```python
from build123d import *

# Parameters (mm, degrees)
SKETCH1_R           = 2.5
BOSS_EXTRUDE1_DEPTH = 61.849
FILLET1_R           = 2
FILLET2_R           = 0.5


with BuildPart() as part:
    # Sketch1 → Boss-Extrude1 (new body, symmetric)
    with BuildSketch(Plane(origin=(0, 0, 0), x_dir=(0, 0, -1), z_dir=(1, 0, 0))):
        Polygon((-2.6, 10), (-2.6, 7.617766953), (-5.85, 7.617766953), (-1.832233047, 3.6), (1.832233047, 3.6), (5.85, 7.617766953), (2.6, 7.617766953), (2.6, 10), (10, 10), (10, 2.6), (7.617766953, 2.6), (7.617766953, 5.85), (3.6, 1.832233047), (3.6, -1.832233047), (7.617766953, -5.85), (7.617766953, -2.6), (10, -2.6), (10, -10), (2.6, -10), (2.6, -7.617766953), (5.85, -7.617766953), (1.832233047, -3.6), (-1.832233047, -3.6), (-5.85, -7.617766953), (-2.6, -7.617766953), (-2.6, -10), (-10, -10), (-10, -2.6), (-7.617766953, -2.6), (-7.617766953, -5.85), (-3.6, -1.832233047), (-3.6, 1.832233047), (-7.617766953, 5.85), (-7.617766953, 2.6), (-10, 2.6), (-10, 10), align=None)
        Circle(SKETCH1_R, mode=Mode.SUBTRACT)
    extrude(amount=BOSS_EXTRUDE1_DEPTH, both=True)

    # Fillet1
    fillet1_edges = [part.edges().sort_by_distance(p)[0] for p in [
        (0, 10, 10),
        (0, 10, -10),
        (0, -10, -10),
        (0, -10, 10),
    ]]
    fillet(fillet1_edges, radius=FILLET1_R)

    # Fillet2
    fillet2_edges = [part.edges().sort_by_distance(p)[0] for p in [
        (0, 10, 2.6),
        (0, 7.617766953, 5.85),
        (0, 3.6, 1.832233047),
        (0, 3.6, -1.832233047),
        (0, 7.617766953, -5.85),
        (0, 10, -2.6),
        (0, 2.6, -10),
        (0, 5.85, -7.617766953),
        (0, 1.832233047, -3.6),
        (0, -1.832233047, -3.6),
        (0, -5.85, -7.617766953),
        (0, -2.6, -10),
        (0, -10, -2.6),
        (0, -7.617766953, -5.85),
        (0, -3.6, -1.832233047),
        (0, -3.6, 1.832233047),
        (0, -7.617766953, 5.85),
        (0, -10, 2.6),
        (0, -2.6, 10),
        (0, -5.85, 7.617766953),
        (0, -1.832233047, 3.6),
        (0, 1.832233047, 3.6),
        (0, 5.85, 7.617766953),
        (0, 2.6, 10),
    ]]
    fillet(fillet2_edges, radius=FILLET2_R)


solid = part.part
```
Part model, mm, in its own coordinate system. A direction names the side the tool comes from. Round coordinates to 2 decimals unless told otherwise and drop trailing zeros. Loops run counter-clockwise (first coordinate to the right, second up) from the corner with the lowest first, then second, coordinate; pieces in that order, holes last.
1. Drill centre lines: line 1 along Y through (x, z) = (-3, 0); line 2 along Z through (x, y) = (39.5, 3.25); line 3 along Z through (x, y) = (-25.5, -5). Where is each one in solid material? Low to high.
Solutions:
line 1: y = -3.6 to -2.5, 2.5 to 3.6
line 2: z = -10 to -7.62, -5.02 to 5.02, 7.62 to 10
line 3: z = -10 to -7.47, -6.77 to -3.23, 3.23 to 6.77, 7.47 to 10
2. Flat gauge pins, fed straight in: pin 1 (3.5 mm diameter, centred on x = 3, z = -0.5, fed in from +Y); pin 2 (2 mm diameter, centred on x = -46, z = -1, fed in from +Y); pin 3 (3.5 mm diameter, centred on x = 7.5, y = 0, fed in from +Z). Where does each tip first touch, or does it go through?
Solutions:
pin 1: stops at y = 4.02
pin 2: stops at y = 3.77
pin 3: stops at z = 3.62
3. 3-axis set-ups, long thin cutter, end or side, ignore diameter. For faces 1 (the face through (1, 0, -3.6)), 2 (the face through (1, 7.618, -4)), 3 (the face through (1, 6, 10)): which of +Z, -Z, +X, -X, +Y, -Y reach the whole face in a straight line?
Solutions:
face 1: -Z, +X, -X
face 2: +X, -X
face 3: +Z, +X, -X, +Y, -Y
4. Slice it at A-A (z = 0). Give the cut face in (x, y), and give its area (3 significant figures).
Solutions:
outline: (-61.85, -3.6) - (61.85, -3.6) - (61.85, -2.5) - (-61.85, -2.5) - close; (-61.85, 2.5) - (61.85, 2.5) - (61.85, 3.6) - (-61.85, 3.6) - close
area: 272 mm2
5. Two-plate mould, pull along Z, no slides. Class faces 4 (the face through (0.87, -3.51, 5.28)), 5 (the face through (0.87, 9.4, 9.43)), 6 (the face through (61.849, 2, 2)): pulls with the +Z half, pulls with the -Z half, needs draft (parallel to the pull), parting line crosses it, or undercut.
Solutions:
face 4: undercut
face 5: pulls with the +Z half
face 6: needs draft
